Source: three-view drawing plus pictorial views. Frame: mm from the lowest corner of the part. Coordinates: 2 decimals unless noted, no trailing zeros. Order: outer loops, then holes, each group sorted by start corner. A loop starts at its lowest first (then second) coordinate and runs counter-clockwise, first axis right, second up. Notation, with made-up numbers: (-4.5, -32.5) -> (42.5, -32.5) arc R20 cw to (42.5, 0.5) -> close; hole circle Ø7 at (48, -26). An arc over 180 degrees is marked (long way). One line per question, with ' | ' between items.
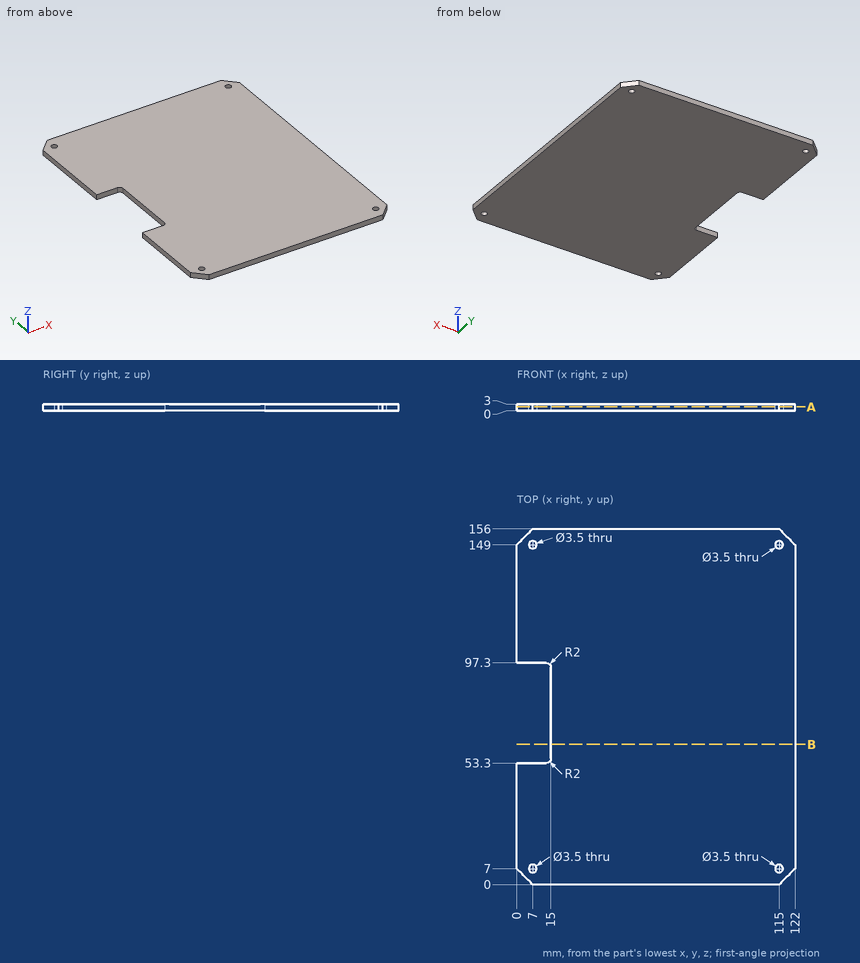
1. Cut plane B-B, the plane y = 61.5. Return loops of the section in (x, z).
Recorded:
outline: (15, 0) -> (122, 0) -> (122, 3) -> (15, 3) -> close
2. Ray query, line 1 (Y direction, x = 115, z = 1.55); line 2 (X direction, y = 7, z = 2.35); line 3 (Y direction, x = 7, z = 2.2). Return the intervals inside material, ascending. Write a range as [from, to].
Recorded:
line 1: y = [0, 5.25], [8.75, 147.25], [150.75, 156] | line 2: x = [0, 5.25], [8.75, 113.25], [116.75, 122] | line 3: y = [0, 5.25], [8.75, 53.3], [97.3, 147.25], [150.75, 156]
3. Pin query (flat end, axial travel): pin 1 Ø0.9 at (x, z) = (9, 2) entering from -Y; pin 2 Ø2 at (x, y) = (115, 149) entering from -Z; pin 3 Ø0.9 at (x, z) = (5.5, 2) entering from +Y; pin 4 Ø1.5 at (y, z) = (74, 2) entering from -X. Return the tip coordinate at first contact, or that it passes through.
Recorded:
pin 1: stops at y = 0 | pin 2: passes through | pin 3: stops at y = 154.95 | pin 4: stops at x = 15
4. Cut plane A-A, the plane z = 1.7. Return loops of the section in (x, y), and give its area (3 significant figures).
Recorded:
outline: (0, 7) -> (7, 0) -> (115, 0) -> (122, 7) -> (122, 149) -> (115, 156) -> (7, 156) -> (0, 149) -> (0, 97.3) -> (13, 97.3) arc R2 cw to (15, 95.3) -> (15, 55.3) arc R2 cw to (13, 53.3) -> (0, 53.3) -> close; hole circle Ø3.5 at (7, 7); hole circle Ø3.5 at (7, 149); hole circle Ø3.5 at (115, 7); hole circle Ø3.5 at (115, 149) | area: 18,200 mm^2
